Model file for the job. Use its own axes, mm. Round coordinates to 2 decimals unless told otherwise and drop trailing zeros. Order: outer loops, then holes, each group sorted by start corner. A loop starts at its lowest first (then second) coordinate and runs counter-clockwise, first axis right, second up. Notation, with made-up numbers: (-6, 86) -> (3, 86) arc R22 ccw to (3, 123) -> close; hole circle Ø9 at (-28.5, 60). An arc over 180 degrees is marked (long way). Put each result on its own line as item: value. Start each with the question number.
Q1. Cut at C-C, the plane y = 13.5. List the corners of the cut face in (x, z).
Q2. Pull direction Y, two halves, no side cores. Call faces 1 (the face through (56.5, -0.7, -725.7)), 2 (the face through (104.7, 9, -368)), 3 (the face through (51, -1, -368)): released by +Y, released by -Y, zero draft, split by the parting line, or undercut.
Q3. Cut at A-A, the plane z = -376.5. List the corners of the cut face in (x, y).
Q4. Cut at B-B, the plane x = 44.5. List the corners of the cut face in (y, z).
Q5. Flat gauge pins, fed straight in: P1, Ø10, axis at y = 6, z = -319, coming from the -X side; P2, Ø1.5, axis at x = 59.5, z = -111, coming from the +Y side; P3, Ø0.5, axis at y = -0.5, z = -14.5, coming from the +X side. Where does each tip first touch, or does it go through?
Q6. Probe L1, parallel to Z at x = 98.7, y = 18.8; L2, parallel to Y at x = 101, z = -364.5; L3, parallel to X at y = 18.75, z = -281.7. List the from-to ranges inside material, lowest first.
from build123d import *

# Parameters (mm, degrees)
SKETCH1_W                    = 105.7
SKETCH1_H                    = 725.7
BASE_FLANGE1_DEPTH           = 1
EDGE_FLANGE1_STRIP_W         = 6
EDGE_FLANGE1_STRIP_H         = 1
EDGE_FLANGE1_STRIP_CUT_DEPTH = 725.7
EDGE_FLANGE1_DEPTH           = 725.7
EDGE_FLANGE2_STRIP_W         = 6
EDGE_FLANGE2_STRIP_H         = 1
EDGE_FLANGE2_STRIP_CUT_DEPTH = 725.7
EDGE_FLANGE2_DEPTH           = 725.7
SKETCH19_R                   = 2.5
CUT_EXTRUDE2_DEPTH           = 10
CUT_EXTRUDE3_START           = -20.5
CUT_EXTRUDE3_DEPTH           = 20.5


# Read off the part's stored shape, not the designer's step: Cut-Extrude3
# Sheet-metal steps are written as plain solids
with BuildPart() as part:
    # Sketch1 → Base-Flange1 (new body)
    with BuildSketch(Plane(origin=(0, 0, 0), x_dir=(1, 0, 0), z_dir=(0, 1, 0))):
        with Locations((52.85, 362.85)):
            Rectangle(SKETCH1_W, SKETCH1_H)
    extrude(amount=-BASE_FLANGE1_DEPTH)

    # Edge-Flange1 strip (across the edge) → Edge-Flange1 strip cut (cut)
    with BuildSketch(Plane(origin=(105.7, 0, 0), x_dir=(-1, 0, 0), z_dir=(0, 0, -1))):
        with Locations((-1, -0.5)):
            Rectangle(EDGE_FLANGE1_STRIP_W, EDGE_FLANGE1_STRIP_H)
    extrude(amount=EDGE_FLANGE1_STRIP_CUT_DEPTH, mode=Mode.SUBTRACT)

    # Edge-Flange1 section (across the edge) → Edge-Flange1 (add)
    with BuildSketch(Plane(origin=(105.7, 0, 0), x_dir=(-1, 0, 0), z_dir=(0, 0, -1))):
        with BuildLine():
            Line((0, 1), (0, 19))
            Line((0, 19), (1, 19))
            Line((1, 19), (1, 1))
            ThreePointArc((1, 1), (1.292893219, 0.292893219), (2, 0))
            Line((2, 0), (2, -1))
            ThreePointArc((2, -1), (0.585786438, -0.414213562), (0, 1))
        make_face()
    extrude(amount=EDGE_FLANGE1_DEPTH)

    # Edge-Flange2 strip (across the edge) → Edge-Flange2 strip cut (cut)
    with BuildSketch(Plane(origin=(104.7, 19, 0), x_dir=(0, -1, 0), z_dir=(0, 0, -1))):
        with Locations((-1, -0.5)):
            Rectangle(EDGE_FLANGE2_STRIP_W, EDGE_FLANGE2_STRIP_H)
    extrude(amount=EDGE_FLANGE2_STRIP_CUT_DEPTH, mode=Mode.SUBTRACT)

    # Edge-Flange2 section (across the edge) → Edge-Flange2 (add)
    with BuildSketch(Plane(origin=(104.7, 19, 0), x_dir=(0, -1, 0), z_dir=(0, 0, -1))):
        with BuildLine():
            Line((0, 1), (0, 12))
            Line((0, 12), (1, 12))
            Line((1, 12), (1, 1))
            ThreePointArc((1, 1), (1.292893219, 0.292893219), (2, 0))
            Line((2, 0), (2, -1))
            ThreePointArc((2, -1), (0.585786438, -0.414213562), (0, 1))
        make_face()
    extrude(amount=EDGE_FLANGE2_DEPTH)

    # Sketch19 → Cut-Extrude2 (cut)
    with BuildSketch(Plane(origin=(0, 19, 0), x_dir=(1, 0, 0), z_dir=(0, 1, 0))):
        with Locations(Location((98.7, 662.7, 0), (0, 0, 180))):
            Circle(SKETCH19_R)
        with Locations(Location((98.7, 617.7, 0), (0, 0, 180))):
            Circle(SKETCH19_R)
        with Locations(Location((98.7, 449.7, 0), (0, 0, 180))):
            Circle(SKETCH19_R)
        with Locations(Location((98.7, 281.7, 0), (0, 0, 180))):
            Circle(SKETCH19_R)
        with Locations(Location((98.7, 113.7, 0), (0, 0, 180))):
            Circle(SKETCH19_R)
        with Locations((98.7, -54.3)):
            Circle(SKETCH19_R)
    extrude(amount=-CUT_EXTRUDE2_DEPTH, mode=Mode.SUBTRACT)

    # Cut-Extrude3 outline → Cut-Extrude3 (cut)
    with BuildSketch(Plane.XY.offset(CUT_EXTRUDE3_START)):
        with BuildLine():
            ThreePointArc((104.7, 1), (104.407106781, 0.292893219), (103.7, 0))
            Line((103.7, 0), (103.7, -1))
            ThreePointArc((103.7, -1), (105.114213562, -0.414213562), (105.7, 1))
            Line((105.7, 1), (105.7, 17))
            ThreePointArc((105.7, 17), (105.114213562, 18.414213562), (103.7, 19))
            Line((103.7, 19), (92.7, 19))
            Line((92.7, 19), (92.7, 18))
            Line((92.7, 18), (103.7, 18))
            ThreePointArc((103.7, 18), (104.407106781, 17.707106781), (104.7, 17))
            Line((104.7, 17), (104.7, 1))
        make_face()
    extrude(amount=CUT_EXTRUDE3_DEPTH, mode=Mode.SUBTRACT)


solid = part.part
Ans:
1. outline: (104.7, -725.7) -> (105.7, -725.7) -> (105.7, -20.5) -> (104.7, -20.5) -> close
2. face 1: zero draft
2. face 2: undercut
2. face 3: released by -Y
3. outline: (0, -1) -> (103.7, -1) arc R2 ccw to (105.7, 1) -> (105.7, 17) arc R2 ccw to (103.7, 19) -> (92.7, 19) -> (92.7, 18) -> (103.7, 18) arc R1 cw to (104.7, 17) -> (104.7, 1) arc R1 cw to (103.7, 0) -> (0, 0) -> close
4. outline: (-1, -725.7) -> (0, -725.7) -> (0, 0) -> (-1, 0) -> close
5. P1: stops at x = 104.7
5. P2: stops at y = 0
5. P3: stops at x = 103.7
6. L1: z = -725.7 to -665.2, -660.2 to -620.2, -615.2 to -452.2, -447.2 to -284.2, -279.2 to -116.2, -111.2 to -20.5
6. L2: y = -1 to 0, 18 to 19
6. L3: x = 92.7 to 96.2, 101.2 to 104.67
